```python
from build123d import *

# Parameters (mm, degrees)
PAD002_DEPTH    = 12
SKETCH005_R     = 5.5
HOLE_DEPTH      = 12.001
SKETCH015_R     = 4
POCKET002_DEPTH = 12.001
SKETCH040_R     = 4
HOLE007_DEPTH   = 622.001


with BuildPart() as side_right_top_part:
    # Sketch002 → Pad002 (new body)
    with BuildSketch(Plane.YZ):
        with BuildLine():
            ThreePointArc((100.076043, 99.923842), (73.635745, 167.771654), (8.210055, 199.738734))
            Line((-66.796185, 205.912919), (8.210055, 199.738734))
            ThreePointArc((-66.796185, 205.912919), (-172.766313, 127.267802), (-108.47912, 12.020766))
            ThreePointArc((-100, 0), (-102.330526, 7.356964), (-108.47912, 12.020766))
            ThreePointArc((-156.643717, -1640.664457), (-114.479942, -820.810119), (-100, 0))
            Line((-156.643717, -1640.664457), (-90.449657, -1649.834344))
            ThreePointArc((-90.449657, -1649.834344), (-85.412451, -1648.162301), (-83.672514, -1643.148141))
            Line((-83.672514, -1643.148141), (-90.302786, -1590.015365))
            ThreePointArc((-83.525643, -1583.329162), (-88.56285, -1585.001205), (-90.302786, -1590.015365))
            Line((-83.525643, -1583.329162), (-17.331583, -1592.49905))
            ThreePointArc((-12.453464, -1600.311408), (-13.065566, -1595.264457), (-17.331583, -1592.49905))
            Line((-12.453464, -1600.311408), (-29.133717, -1651.191872))
            ThreePointArc((-29.133717, -1651.191872), (-28.521615, -1656.238824), (-24.255598, -1659.004231))
            Line((-24.255598, -1659.004231), (41.938462, -1668.174118))
            ThreePointArc((41.938462, -1668.174118), (85.162756, -834.581071), (100, 0))
            Line((100, 0), (100.076043, 99.923842))
        make_face()
    extrude(amount=PAD002_DEPTH)

    # Sketch005 → Hole (cut, through all)
    with BuildSketch(Plane.YZ):
        with Locations((0, 100)):
            Circle(SKETCH005_R)
        with Locations((-75, 106.25)):
            Circle(SKETCH005_R)
        Circle(SKETCH005_R)
    extrude(amount=HOLE_DEPTH, mode=Mode.SUBTRACT)

    # Sketch015 → Pocket002 (cut, through all)
    with BuildSketch(Plane.YZ):
        with Locations((-0.303341, -120.666401)):
            Circle(SKETCH015_R)
        with Locations((-0.669999, -179.331911)):
            Circle(SKETCH015_R)
        with Locations((-29.495132, -1189.859798)):
            Circle(SKETCH015_R)
        with Locations((-32.518295, -1249.351095)):
            Circle(SKETCH015_R)
        with Locations((-130.873609, -2506.378514)):
            Circle(SKETCH015_R)
        with Locations((-136.971781, -2564.727371)):
            Circle(SKETCH015_R)
        with BuildLine():
            ThreePointArc((-63.5924, -1210.755644), (-69.621614, -1215.669765), (-64.707493, -1221.698978))
            Line((-64.707493, -1221.698978), (1.615745, -1228.457117))
            ThreePointArc((1.615745, -1228.457117), (7.644959, -1223.542997), (2.730838, -1217.513783))
            Line((2.730838, -1217.513783), (-63.5924, -1210.755644))
        make_face()
        with BuildLine():
            ThreePointArc((-33.802079, -144.499268), (-39.302079, -149.999268), (-33.802079, -155.499268))
            Line((-33.802079, -155.499268), (32.864588, -155.499268))
            ThreePointArc((32.864588, -155.499268), (38.364588, -149.999268), (32.864588, -144.499268))
            Line((32.864588, -144.499268), (-33.802079, -144.499268))
        make_face()
        with BuildLine():
            ThreePointArc((-165.386078, -2523.207318), (-171.913956, -2527.436597), (-167.684677, -2533.964476))
            Line((-167.684677, -2533.964476), (-102.489783, -2547.895382))
            ThreePointArc((-102.489783, -2547.895382), (-95.961904, -2543.666103), (-100.191183, -2537.138225))
            Line((-100.191183, -2537.138225), (-165.386078, -2523.207318))
        make_face()
        with BuildLine():
            ThreePointArc((-307.201152, -3631.252582), (-314.086519, -3634.870829), (-310.468272, -3641.756197))
            Line((-310.468272, -3641.756197), (-246.81, -3661.556925))
            ThreePointArc((-246.81, -3661.556925), (-239.924632, -3657.938678), (-243.542879, -3651.05331))
            Line((-243.542879, -3651.05331), (-307.201152, -3631.252582))
        make_face()
        with BuildLine():
            ThreePointArc((-498.714671, -4731.898869), (-505.894975, -4734.889394), (-502.90445, -4742.069697))
            Line((-502.90445, -4742.069697), (-441.263063, -4767.462292))
            ThreePointArc((-441.263063, -4767.462292), (-434.082759, -4764.471767), (-437.073284, -4757.291463))
            Line((-437.073284, -4757.291463), (-498.714671, -4731.898869))
        make_face()
    extrude(amount=POCKET002_DEPTH, mode=Mode.SUBTRACT)

    # Sketch040 (on Face1 of ShapeBinder) → Hole007 (cut, through all)
    with BuildSketch(Plane(origin=(-610, 0, 0), x_dir=(0, -1, 0), z_dir=(-1, 0, 0))):
        with Locations((-32.147032, -1454.701534)):
            Circle(SKETCH040_R)
        with Locations((-2.949201, -1878.284217)):
            Circle(SKETCH040_R)
        with Locations((-76.414195, -37.446092)):
            Circle(SKETCH040_R)
    extrude(amount=-HOLE007_DEPTH, mode=Mode.SUBTRACT)


with BuildPart() as side_right_top_part_1:
    # Body003 placement: moved
    add(side_right_top_part.part.moved(Location((610, 0, 0))))


with BuildPart() as side_left_top_part:
    # Part__Mirroring: instance of side_right_top_part
    add(side_right_top_part_1.part.mirror(Plane(origin=(-0.000122, -37.441761, -731.130615), x_dir=(0, -1, 0), z_dir=(1, 0, 0))))


solid = side_left_top_part.part
```
CAD build for the part. Positions are in the model's coordinates, mm. Round coordinates to 2 decimals unless told otherwise and drop trailing zeros. Loops run counter-clockwise (first coordinate to the right, second up) from the corner with the lowest first, then second, coordinate; pieces in that order, holes last. Notation, with made-up numbers: (50.5, 83) - (64.5, 83) arc R20 cw to (64.5, 120) - close; hole circle Ø10 at (21.5, -1.5). An arc over 180 degrees is marked (long way). Return JSON: item names as keys, results as strings. Group by question number.
Q1. Drill centre lines: line 1 along Y through (x, z) = (-613.5, 108); line 2 along Y through (x, z) = (-614.25, 0); line 3 along Z through (x, y) = (-621, 30). Where is each one in solid material? Low to high. Write a range as [from, to].
Q2. Band-saw the part on C-C on z = -1049. Give the cut face in (x, y).
Q3. Band-saw the part on A-A on x = -615. Give the number of separate pieces and of enclosed holes in the cut face, plus the area to 3 significant figures.
Q4. Two-plate mould, pull along Z, no slides. Class faces 1 (the face through (-615.92, -114.88, -832.3)), 2 (the face through (-610, -9, -718)): +Z half, -Z half, draft (parallel to the pull), parting line (faces both ways), or undercut.
Q5. Band-saw the part on B-B on z = -261. Give the cut face in (x, y), plus the area to 3 significant figures.
Q6. Flat gauge pins, fed straight in: pin 1 Ø12.5 at (y, z) = (-75, 106.25) entering from -X; pin 2 Ø1 at (x, y) = (-611.5, 8.5) entering from -Z; pin 3 Ø1 at (x, z) = (-611.5, -844) entering from +Y; pin 4 Ø6 at (x, y) = (-616.5, 10.5) entering from -Z. Where does each tip first touch, or does it go through?
Solutions:
{
 "1": {"line 1": "y = [-174.98, -80.21], [-69.79, 99.76]", "line 2": "y = [-100, -5.5], [5.5, 100]", "line 3": "z = [-1666.52, -1458.08], [-1451.33, -155.5], [-144.5, 195.47]"},
 "2": {"outline": "(-622, -123.43) - (-610, -123.43) - (-610, 76.76) - (-622, 76.76) - close"},
 "3": {"separate pieces": "1", "enclosed holes": "11", "area": "373,000 mm^2"},
 "4": {"face 1": "undercut", "face 2": "draft"},
 "5": {"outline": "(-622, -101.6) - (-610, -101.6) - (-610, 98.41) - (-622, 98.41) - close", "area": "2,400 mm^2"},
 "6": {"pin 1": "stops at x = -622", "pin 2": "stops at z = -1663.61", "pin 3": "stops at y = 84.85", "pin 4": "stops at z = -1664.23"}
}
